The listing builds one solid part. Answer for the finished solid, in the listing's coordinates (mm). A direction names the side the tool comes from. Coordinates: 2 decimals unless noted, no trailing zeros. Loops run counter-clockwise (first coordinate to the right, second up) from the corner with the lowest first, then second, coordinate; pieces in that order, holes last. Notation, with made-up numbers: M 0.5,71 L 23.5,71 A17 ccw 23.5,75 Z; hole C 39.25,-9 d5. An arc over 180 degrees is marked long. Answer as a JSON object with one key per item and string values. Group by question number.
1. Straight lines are drawn through the part: L1, parallel to Y at x = 27, z = 3; L2, parallel to Y at x = 21, z = 2.5; L3, parallel to X at y = 10.75, z = 0.3. For each, find the intervals that lie inside material, in ascending order.
2. A cutting plane is placed at A-A on y = 6. Give the vertices of the cut face in (x, z) (3 decimals), and give its area (3 significant figures).
3. Given pin 1 (0.9 mm diameter, centred on y = 8, z = 1.5, fed in from +X); pin 2 (0.5 mm diameter, centred on y = 6, z = 2, fed in from +X), each flat-ended and moving along its own axis, determine where each tip first touches the part or whether it passes through.
4. For faces 1 (the face through (15, 20.392, 2)), 2 (the face through (21, 5.669, 2)), 3 (the face through (25.759, 5, 2)), determine the directions among +Z, -Z, +X, -X, +Y, -Y from which every point of the face is accessible in a straight line to the end or side of a thin tool.
5. Determine the mould class of faces 4 (the face through (14, 9, 0)), 5 (the face through (14, -2.608, 2)), 6 (the face through (20.434, 7, 2)), 7 (the face through (22.434, 11, 2)) for opening direction Y: released by +Y, released by -Y, zero draft, split by the parting line, or undercut.
6. A cutting plane is placed at B-B on z = 1.55. Give the vertices of the cut face in (x, y).
from build123d import *

# Parameters (mm, degrees)
F0_R     = 0.75
F0_W     = 3.175
F0_H     = 6
F1_DEPTH = 3.175


# Not quite as in the source:
# - a length typed as a fraction of an inch, garbled in the dataset ("3 / 203.2 mm" for 3/8 in), is restored


with BuildPart() as f1:
    # F0 (on Top) → F1 (new body)
    with BuildSketch(Plane.XY):
        Polygon((18.934352152, 7.3924250901), (18.934352152, 10.3924250901), (20.434352152, 10.3924250901), (20.434352152, 12.1162086725), (22.434352152, 12.1162086725), (22.434352152, 10.3924250901), (25.759352152, 10.3924250901), (25.759352152, 14.3924250901), (25.759352152, 20.3924250901), (0.434352152, 20.3924250901), (0.434352152, -2.6075749099), (25.759352152, -2.6075749099), (25.759352152, 3.3924250901), (25.759352152, 7.3924250901), (22.434352152, 7.3924250901), (22.434352152, 5.6686415076), (20.434352152, 5.6686415076), (20.434352152, 7.3924250901), align=None)
        with Locations((4.184352152, 3.9924250901)):
            Circle(F0_R, mode=Mode.SUBTRACT)
        with BuildLine():
            ThreePointArc((14.934352152, 3.9924250901), (13.6540220662, 3.4620950042), (14.184352152, 4.7424250901))
            ThreePointArc((14.184352152, 4.7424250901), (14.7146822379, 4.522755176), (14.934352152, 3.9924250901))
        make_face(mode=Mode.SUBTRACT)
        with Locations((4.184352152, 13.7924250901)):
            Circle(F0_R, mode=Mode.SUBTRACT)
        with BuildLine():
            ThreePointArc((14.184352152, 13.0424250901), (13.6540220662, 14.322755176), (14.934352152, 13.7924250901))
            ThreePointArc((14.934352152, 13.7924250901), (14.7146822379, 13.2620950042), (14.184352152, 13.0424250901))
        make_face(mode=Mode.SUBTRACT)
        with Locations((27.346852152, 17.3924250901)):
            Rectangle(F0_W, F0_H)
        with Locations((27.346852152, 0.3924250901)):
            Rectangle(F0_W, F0_H)
    extrude(amount=F1_DEPTH)


solid = f1.part
From the geometry:
{
 "1": {"L1": "y = -2.61 to 3.39, 14.39 to 20.39", "L2": "y = -2.61 to 5.67, 12.12 to 20.39", "L3": "x = 0.43 to 20.43, 22.43 to 25.76"},
 "2": {"outline": "M 0.434,0 L 20.434,0 L 20.434,3.175 L 0.434,3.175 Z; M 22.434,0 L 25.759,0 L 25.759,3.175 L 22.434,3.175 Z", "area": "74.1 mm²"},
 "3": {"pin 1": "stops at x = 18.93", "pin 2": "stops at x = 25.76"},
 "4": {"face 1": "+Z, -Z, +X, -X, +Y", "face 2": "+Z, -Z", "face 3": "+Z, -Z, +X"},
 "5": {"face 4": "zero draft", "face 5": "released by -Y", "face 6": "undercut", "face 7": "undercut"},
 "6": {"outline": "M 0.43,-2.61 L 28.93,-2.61 L 28.93,3.39 L 25.76,3.39 L 25.76,7.39 L 22.43,7.39 L 22.43,5.67 L 20.43,5.67 L 20.43,7.39 L 18.93,7.39 L 18.93,10.39 L 20.43,10.39 L 20.43,12.12 L 22.43,12.12 L 22.43,10.39 L 25.76,10.39 L 25.76,14.39 L 28.93,14.39 L 28.93,20.39 L 0.43,20.39 Z; hole C 4.18,3.99 d1.5; hole C 4.18,13.79 d1.5; hole C 14.18,3.99 d1.5; hole C 14.18,13.79 d1.5"}
}
